Autodesk Inventor part; units mm, degrees
ref_plane "YZ Plane" through (0, 0, 0) normal (1, 0, 0) x (0, 1, 0)
ref_plane "XZ Plane" through (0, 0, 0) normal (0, 1, 0) x (-1, 0, 0)
ref_plane "XY Plane" through (0, 0, 0) normal (0, 0, 1) x (1, 0, 0)
sketch "스케치1" plane through (0, 0, 0) normal (0, 0, 1) x (1, 0, 0)
  line L0 (0, 0) -> (9, 0)
  line L1 (9, 0) -> (9, 10.5)
  line L2 (9, 10.5) -> (0, 10.5)
  line L3 (0, 10.5) -> (0, 0)
  line L4 (-1.5, 12) -> (10.5, 12)
  line L5 (10.5, 12) -> (10.5, -1.5)
  line L6 (10.5, -1.5) -> (-1.5, -1.5)
  line L7 (-1.5, -1.5) -> (-1.5, 12)
  line L8 (0, 0) -> (0, -1.5)
  line L9 (9, 0) -> (9, -1.5)
  line L10 (0, 0) -> (-1.5, 0)
  line L11 (9, 0) -> (10.5, 0)
  dimension "d0" = 9
  dimension "d1" = 10.5
  dimension "d2" = 1.5
extrude "돌출1" add sketch "스케치1" along normal blind 20 contours L10 L7 L4 L5 L11 L1 L2 L3 | L8 L6 L7 L10 | L11 L5 L6 L9
sketch "스케치2" plane through (-1.5, -1.5, 0) normal (0, -1, 0) x (1, 0, 0)
  line L0 (0, 0) -> (1.5, 0)
  line L1 (1.5, 0) -> (1.5, 20)
  line L2 (0, 20) -> (1.5, 20)
  line L3 (0, 0) -> (0, 20)
  line L4 (1.5, 5) -> (0, 5)
  line L5 (0, 5) -> (0, 5.8)
  line L6 (0, 5.8) -> (1.5, 5.8)
  line L7 (1.5, 5.8) -> (1.5, 5)
  point P0 (1.5, 0)
  point P1 (1.5, 5.8)
  point P2 (0, 5)
  dimension "d5" = 0.8
  dimension "d6" = 5
extrude "돌출2" cut sketch "스케치2" against normal blind 8 contours L3 L6 L1 L4
fillet "모깎기1" radius 2 2 edges at (-1.5, 12, 10) (10.5, 12, 10)
sketch "스케치5" plane through (0, 10.5, 0) normal (0, -1, 0) x (1, 0, 0)
  line L0 (0, 0) -> (9, 0)
  line L1 (9, 0) -> (9, 20)
  line L2 (0, 20) -> (9, 20)
  line L3 (0, 0) -> (0, 20)
  line L4 (9, 17.5) -> (7, 17.5)
  line L5 (7, 17.5) -> (7, 20)
  line L6 (8.5, 20) -> (0.5, 20)
  point P0 (0, 0)
  dimension "d21" = 2.5
  dimension "d22" = 2
extrude "돌출5" add sketch "스케치5" along normal blind 5 contours L4 L5 L2 L1
sketch "스케치7" plane through (0, 0, 20) normal (0, 0, 1) x (1, 0, 0)
  arc A0 (10.5, 10) -> (8.5, 12) centre (8.5, 10) ccw
  line L0 (8.5, 12) -> (0.5, 12)
  arc A1 (0.5, 12) -> (-1.5, 10) centre (0.5, 10) ccw
  line L1 (-1.5, 10) -> (-1.5, -1.5)
  line L2 (-1.5, -1.5) -> (0, -1.5)
  line L3 (0, -1.5) -> (0, 10.5)
  line L4 (0, 10.5) -> (7, 10.5)
  line L5 (7, 10.5) -> (7, 5.5)
  line L6 (9, 5.5) -> (7, 5.5)
  line L7 (9, 5.5) -> (9, -1.5)
  line L8 (9, -1.5) -> (10.5, -1.5)
  line L9 (10.5, -1.5) -> (10.5, 10)
  line L10 (0, 10.5) -> (9, 10.5)
  line L11 (7, 10.5) -> (7, 12)
  line L12 (8.5, 12) -> (0.5, 12)
  point P0 (0, 0)
extrude "돌출6" cut sketch "스케치7" against normal blind 1.5 contours L11 L4 L3 L2 L1 A1 L0
properties part number "_3D 인쇄"
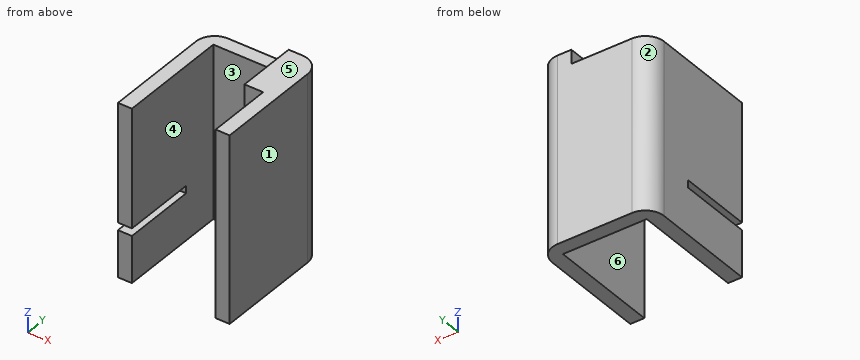
The model under review builds one solid part; all positions refer to its coordinate system, in mm. Face numbers are marked on the shaded views. A direction names the side the tool comes from. Round coordinates to 2 decimals unless told otherwise and drop trailing zeros. Order: outer loops, then holes, each group sorted by start corner. A loop starts at its lowest first (then second) coordinate and runs counter-clockwise, first axis right, second up.
(1) Tool access review of the marked faces 4, 5 and 6: name each direction out of +Z, -Z, +X, -X, +Y, -Y from which nothing blocks a thin tool from reaching the whole face with its end or side.
Working result:
face 4: +Z, -Z, -Y
face 5: +Z, +X, -X, +Y, -Y
face 6: -Z, -Y
(2) Take a section at C-C, the plane z = 18.75. State the section outline as (x, y) points.
Working result:
outline: (7, 5.5) - (9, 5.5) - (9, -1.5) - (10.5, -1.5) - (10.5, 10) arc R2 ccw to (8.5, 12) - (7, 12) - close
(3) Wall thickness on L1, parallel to X at y = 0.5, z = 6; L2, parallel to Y at x = 4.75, z = 4; L3, parallel to Y at x = 9.5, z = 11: over which ranges is each line inside the solid? List them lowest first.
Working result:
L1: x = -1.5 to 0, 9 to 10.5
L2: y = 10.5 to 12
L3: y = -1.5 to 11.73
(4) Take a section at A-A, the plane y = 2.75. State the section outline as (x, z) points.
Working result:
outline: (-1.5, 0) - (0, 0) - (0, 5) - (-1.5, 5) - close; (-1.5, 5.8) - (0, 5.8) - (0, 18.5) - (-1.5, 18.5) - close; (9, 0) - (10.5, 0) - (10.5, 20) - (9, 20) - close
(5) Take a section at B-B, the plane y = 6.75. State the section outline as (x, z) points.
Working result:
outline: (-1.5, 0) - (0, 0) - (0, 18.5) - (-1.5, 18.5) - close; (7, 17.5) - (9, 17.5) - (9, 0) - (10.5, 0) - (10.5, 20) - (7, 20) - close
(6) Mouldability with a two-part tool opening along X and no side actions: class the marked faces 1, 2 and 3 as released by +X, released by -X, zero draft, split by the parting line, or undercut.
Working result:
face 1: released by +X
face 2: released by -X
face 3: undercut
(7) Take a section at D-D, the plane x = -0.25. State the section outline as (y, z) points, plus the area to 3 significant figures.
Working result:
outline: (-1.5, 0) - (11.85, 0) - (11.85, 18.5) - (-1.5, 18.5) - (-1.5, 5.8) - (6.5, 5.8) - (6.5, 5) - (-1.5, 5) - close
area: 241 mm2
(8) For P1, Ø0.8, axis at x = -0.5, y = 2.5, coming from the +Z side; P2, Ø1.5, axis at x = 3, z = 17.5, coming from the -Y side; P3, Ø0.6, axis at x = 8, y = 8.5, coming from the -Z side, all flat-tipped, find the tip position at first contact; note any pin that passes through.
Working result:
P1: stops at z = 18.5
P2: stops at y = 10.5
P3: stops at z = 17.5
